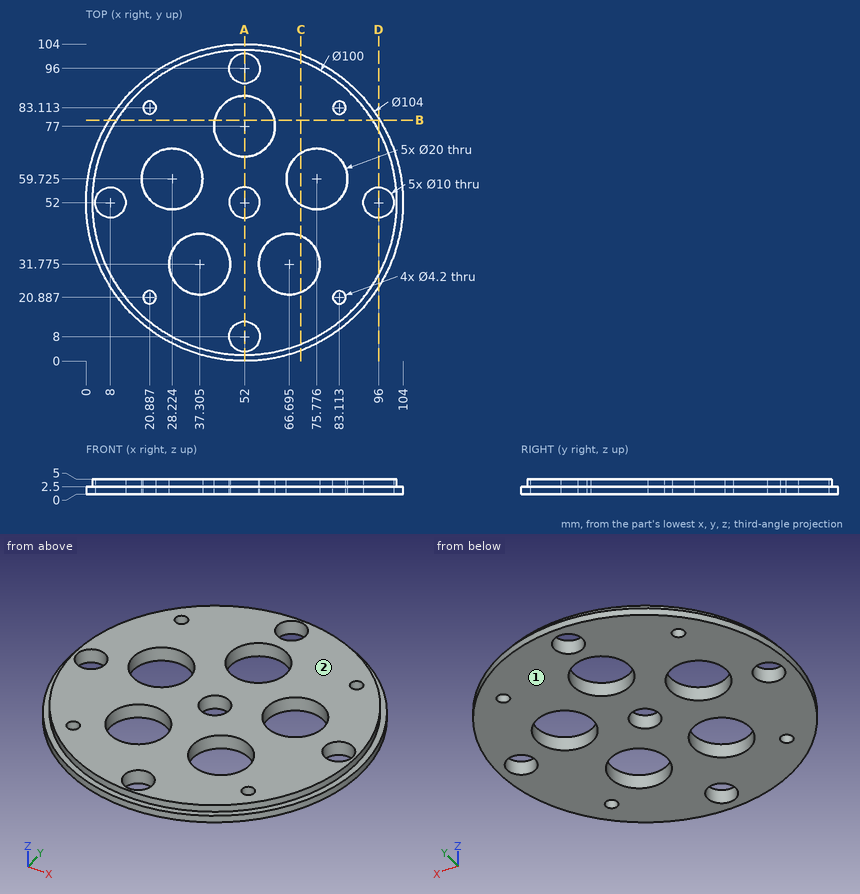
Source: three-view drawing plus pictorial views. Frame: mm from the lowest corner of the part. Coordinates: 2 decimals unless noted, no trailing zeros. Loops run counter-clockwise (first coordinate to the right, second up) from the corner with the lowest first, then second, coordinate; pieces in that order, holes last. Notation, with made-up numbers: (0, 60) - (28, 60) arc R22 cw to (28, 85) - close; hole circle Ø11 at (66, 47.5). An arc over 180 degrees is marked (long way). One line per item, written item: value. Start each with the question number.
1. Section A-A (x = 52). Return the cut outline in (y, z).
2. Section B-B (y = 79). Return the cut outline in (x, z).
3. Contact query for flat-ended pins moving along their axis: P1, Ø23, axis at x = 52, y = 77, coming from the -Z side; P2, Ø3.5, axis at x = 20.89, y = 83.11, coming from the -Z side; P3, Ø1, axis at y = 27, z = 3.5, coming from the +X side. Output: stop coordinate, or through.
4. Section D-D (x = 96). Return the cut outline in (y, z).
5. Ray query, L1, parallel to X at y = 58, z = 3.2; L2, parallel to Y at x = 47.5, z = 4.35 (1 decimal); L3, parallel to Y at x = 48.5, z = 0.6. Return the intervals inside material, ascending.
6. Section C-C (x = 70.5). Return the cut outline in (y, z), and give its area (3 significant figures).
7. Mould query, pull axis Z, two halves, no side actions, for the marked faces 1 and 2. Classes: pulls with the +Z half, pulls with the -Z half, needs draft (parallel to the pull), parting line crosses it, or undercut.
Verdict:
1. outline: (0, 0) - (3, 0) - (3, 5) - (2, 5) - (2, 2.5) - (0, 2.5) - close; (13, 0) - (47, 0) - (47, 5) - (13, 5) - close; (57, 0) - (67, 0) - (67, 5) - (57, 5) - close; (87, 0) - (91, 0) - (91, 5) - (87, 5) - close; (101, 0) - (104, 0) - (104, 2.5) - (102, 2.5) - (102, 5) - (101, 5) - close
2. outline: (7.56, 0) - (42.2, 0) - (42.2, 5) - (9.92, 5) - (9.92, 2.5) - (7.56, 2.5) - close; (61.8, 0) - (96.44, 0) - (96.44, 2.5) - (94.08, 2.5) - (94.08, 5) - (61.8, 5) - close
3. P1: stops at z = 0
3. P2: passes through
3. P3: stops at x = 95.59
4. outline: (24.29, 0) - (47, 0) - (47, 5) - (28.25, 5) - (28.25, 2.5) - (24.29, 2.5) - close; (57, 0) - (79.71, 0) - (79.71, 2.5) - (75.75, 2.5) - (75.75, 5) - (57, 5) - close
5. L1: x = 2.36 to 18.37, 38.07 to 65.93, 85.63 to 101.64
5. L2: y = 2.2 to 5.8, 10.2 to 49.8, 54.2 to 68.1, 85.9 to 93.8, 98.2 to 101.8
5. L3: y = 0.12 to 4.43, 11.57 to 48.43, 55.57 to 67.63, 86.37 to 92.43, 99.57 to 103.88
6. outline: (3.4, 0) - (22.53, 0) - (22.53, 5) - (5.55, 5) - (5.55, 2.5) - (3.4, 2.5) - close; (41.02, 0) - (51.23, 0) - (51.23, 5) - (41.02, 5) - close; (68.22, 0) - (100.6, 0) - (100.6, 2.5) - (98.45, 2.5) - (98.45, 5) - (68.22, 5) - close
6. area: 298 mm2
7. face 1: pulls with the -Z half
7. face 2: pulls with the +Z half
